from build123d import *

# Parameters (mm, degrees)
SKETCH1_W           = 45.72
SKETCH1_H           = 6.35
BOSS_EXTRUDE1_DEPTH = 1.5875
SKETCH4_W           = 6.35
SKETCH4_H           = 3.175
CUT_EXTRUDE1_DEPTH  = 3.175
SKETCH5_W           = 2.2225
SKETCH5_H           = 3.175
BOSS_EXTRUDE3_DEPTH = 3.175
SKETCH3_R           = 1.25
CUT_EXTRUDE2_DEPTH  = 6.985


with BuildPart() as part:
    # Sketch1 → Boss-Extrude1 (new body, symmetric)
    with BuildSketch(Plane(origin=(0, 0, 0), x_dir=(1, 0, 0), z_dir=(0, 1, 0))):
        Rectangle(SKETCH1_W, SKETCH1_H)
    extrude(amount=BOSS_EXTRUDE1_DEPTH, both=True)

    # Sketch4 → Cut-Extrude1 (cut)
    with BuildSketch(Plane.XY.offset(3.175)):
        with Locations((-6.985, 0)):
            Rectangle(SKETCH4_W, SKETCH4_H)
    extrude(amount=-CUT_EXTRUDE1_DEPTH, mode=Mode.SUBTRACT)

    # Sketch5 → Boss-Extrude3 (add)
    with BuildSketch(Plane(origin=(0, 1.5875, 0), x_dir=(1, 0, 0), z_dir=(0, 1, 0))):
        with Locations((-5.87375, 1.5875)):
            Rectangle(SKETCH5_W, SKETCH5_H)
    extrude(amount=BOSS_EXTRUDE3_DEPTH)

    # Sketch3 → Cut-Extrude2 (cut)
    with BuildSketch(Plane.ZY.offset(22.86)):
        Circle(SKETCH3_R)
    cut_extrude2 = extrude(amount=-CUT_EXTRUDE2_DEPTH, mode=Mode.SUBTRACT)

    # Mirror1: Cut-Extrude2 across plane
    add(cut_extrude2.mirror(Plane(origin=(0, 0, 0), x_dir=(0, 0, 1), z_dir=(1, 0, 0))), mode=Mode.SUBTRACT)


solid = part.part
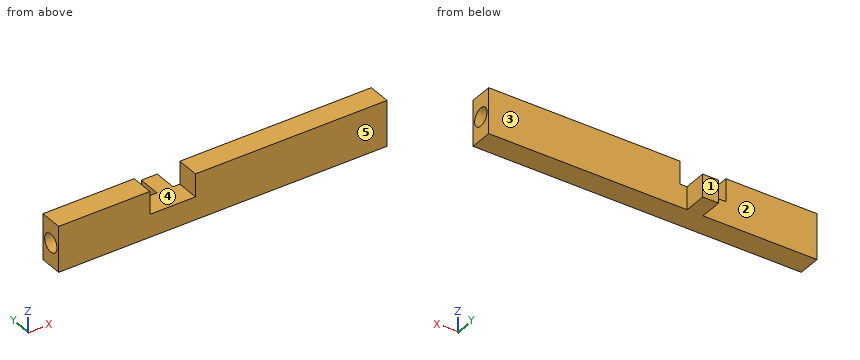
Source: CAD feature listing. Evaluate the final solid. Frame: model axes, mm. Face numbers are marked on the shaded views. A direction names the side the tool comes from. Give positions to 0.01 mm unless a question says otherwise; leave off trailing zeros. Order: outer loops, then holes, each group sorted by start corner. A loop starts at its lowest first (then second) coordinate and runs counter-clockwise, first axis right, second up. Notation, with made-up numbers: (-4.5, -4.5) -> (44.5, -4.5) arc R27 ccw to (44.5, 26.5) -> close; hole circle Ø2 at (54, 43.5). An arc over 180 degrees is marked (long way). Use a Markdown table: item, result.
1) Ray query, line 1 along X through (y, z) = (-0.25, 1.5); line 2 along X through (y, z) = (-0.25, 1) (3 decimals); line 3 along Y through (x, z) = (20.25, 0). Return the intervals inside material, ascending. Write a range as [from, to].
Answer list:
| item | result |
|---|---|
| line 1 | [-22.86, -10.16], [-3.81, 22.86] |
| line 2 | [-15.875, -10.16], [-3.81, 15.875] |
| line 3 | [-1.59, -1.25], [1.25, 1.59] |
2) Section query D-D, the plane z = -0.75. Return the cut outline in (x, y) (1 decimal).
Answer list:
| item | result |
|---|---|
| outline | (-22.9, -1.6) -> (22.9, -1.6) -> (22.9, -1) -> (15.9, -1) -> (15.9, 1) -> (22.9, 1) -> (22.9, 1.6) -> (-4.8, 1.6) -> (-4.8, 4.8) -> (-7, 4.8) -> (-7, 1.6) -> (-22.9, 1.6) -> (-22.9, 1) -> (-15.9, 1) -> (-15.9, -1) -> (-22.9, -1) -> close |
3) Reachability of the marked faces 1, 2 and 3 from +Z, -Z, +X, -X, +Y, -Y: full face, straight path, thin tool, end or side. Return the list, or none.
Answer list:
| item | result |
|---|---|
| face 1 | +Z, -Z, +X, -X, +Y |
| face 2 | +Z, -Z, -X, +Y |
| face 3 | +Z, -Z, +X, +Y |
4) Section query A-A, the plane z = 2.25. Return the cut outline in (x, y).
Answer list:
| item | result |
|---|---|
| outline | (-22.86, -1.59) -> (-10.16, -1.59) -> (-10.16, 1.59) -> (-22.86, 1.59) -> close; (-3.81, -1.59) -> (22.86, -1.59) -> (22.86, 1.59) -> (-3.81, 1.59) -> close |
5) Contact query for flat-ended pins moving along their axis: P1, Ø2, axis at y = 0.5, z = 0, coming from the +X side; P2, Ø2.5, axis at y = 3, z = -2, coming from the +X side; P3, Ø1.5, axis at y = 0, z = 0, coming from the -X side (3 decimals); P4, Ø1.9, axis at x = 14.5, z = -1.5, coming from the +Y side. Output: stop coordinate, or through.
Answer list:
| item | result |
|---|---|
| P1 | x = 22.86 |
| P2 | x = -4.76 |
| P3 | x = -15.875 |
| P4 | y = 1.59 |
6) Mould query, pull axis X, two halves, no side actions, for the marked faces 4 and 5. Classes: +X half, -X half, draft (parallel to the pull), parting line (faces both ways), or undercut.
Answer list:
| item | result |
|---|---|
| face 4 | undercut |
| face 5 | draft |
7) Section query B-B, the plane y = 0. Return the cut outline in (x, z) (3 decimals), then the cut area to 3 significant figures.
Answer list:
| item | result |
|---|---|
| outline | (-22.86, -3.175) -> (22.86, -3.175) -> (22.86, -1.25) -> (15.875, -1.25) -> (15.875, 1.25) -> (22.86, 1.25) -> (22.86, 3.175) -> (-3.81, 3.175) -> (-3.81, 0) -> (-10.16, 0) -> (-10.16, 3.175) -> (-22.86, 3.175) -> (-22.86, 1.25) -> (-15.875, 1.25) -> (-15.875, -1.25) -> (-22.86, -1.25) -> close |
| area | 235 mm² |
